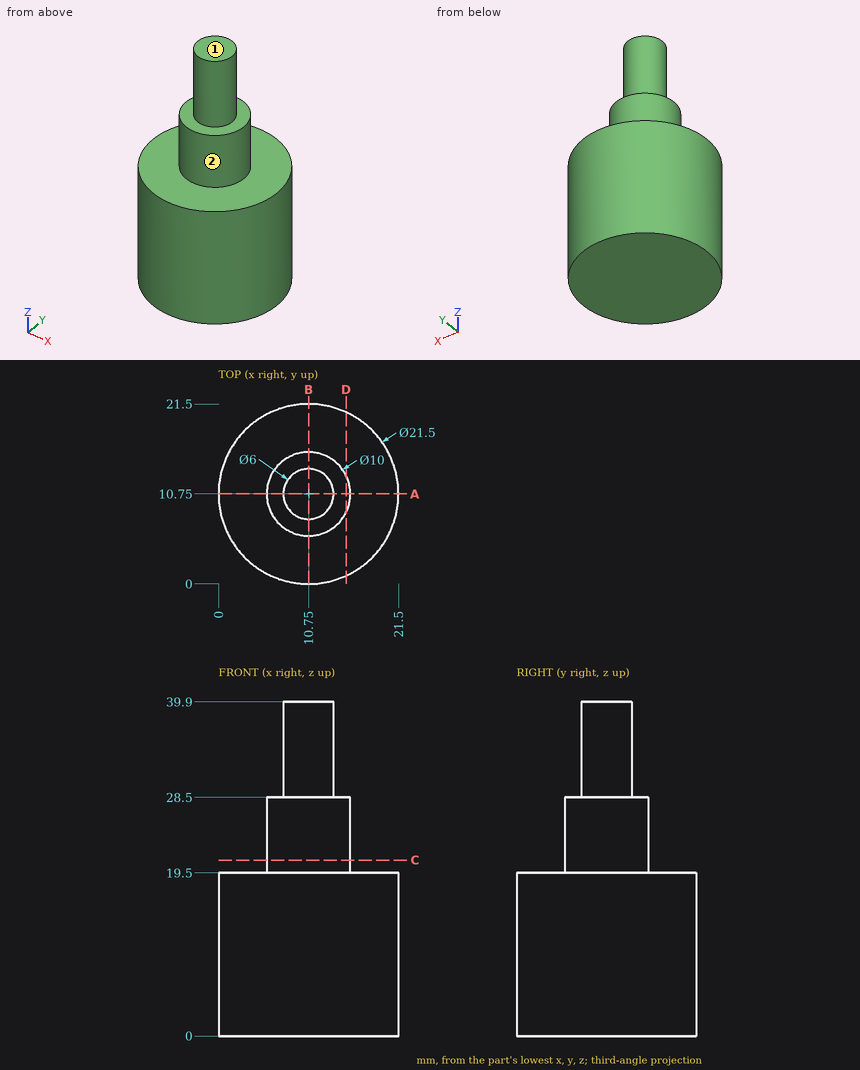
Design review of the part shown in the three views and the two pictorial views. Dimensions are in mm from the part's minimum x, y and z. A direction names the side the tool comes from. Give positions to 0.01 mm unless a question says otherwise; leave off trailing zeros. Loops run counter-clockwise (first coordinate to the right, second up) from the corner with the lowest first, then second, coordinate; pieces in that order, holes last. Notation, with made-up numbers: M 55,51.25 L 90,51.25 A24 ccw 90,65.25 Z; hole C -7,-16 d2. An arc over 180 degrees is marked long. Put each result on its own line as item: value. Start each with the question number.
(1) Add section D-D, the plane x = 15.25. Write out the cut boundary in (y, z).
(2) Wall thickness on L1, parallel to Z at x = 20.5, y = 10.75; L2, parallel to Z at x = 13.5, y = 8.5; L3, parallel to Y at x = 10.75, z = 38: over which ranges is each line inside the solid? List them lowest first.
(3) Add section A-A, the plane y = 10.75. Write out the cut boundary in (x, z), then the cut area to 3 significant figures.
(4) Machinability: for the marked faces 1 and 2, which of the approach directions +Z, -Z, +X, -X, +Y, -Y give a long, thin tool a straight path to every point of the face, cutting with its end or side? Answer none if there is none.
(5) Add section C-C, the plane z = 21. Write out the cut boundary in (x, y), then the cut area to 3 significant figures.
(6) For pin 1 (3 mm diameter, centred on x = 17, z = 5, fed in from +Y); pin 2 (2 mm diameter, centred on x = 5, y = 13.5, fed in from +Z); pin 3 (1 mm diameter, centred on x = 7, z = 19, fed in from +Y); pin 4 (5 mm diameter, centred on y = 19, z = 28.5, fed in from -X), all flat-tipped, find the tip position at first contact; note any pin that passes through.
Result:
1. outline: M 0.99,0 L 20.51,0 L 20.51,19.5 L 12.93,19.5 L 12.93,28.5 L 8.57,28.5 L 8.57,19.5 L 0.99,19.5 Z
2. L1: z = 0 to 19.5
2. L2: z = 0 to 28.5
2. L3: y = 7.75 to 13.75
3. outline: M 0,0 L 21.5,0 L 21.5,19.5 L 15.75,19.5 L 15.75,28.5 L 13.75,28.5 L 13.75,39.9 L 7.75,39.9 L 7.75,28.5 L 5.75,28.5 L 5.75,19.5 L 0,19.5 Z
3. area: 578 mm^2
4. face 1: +Z, +X, -X, +Y, -Y
4. face 2: +Z
5. outline: C 10.75,10.75 d10
5. area: 78.5 mm^2
6. pin 1: stops at y = 20.39
6. pin 2: stops at z = 19.5
6. pin 3: stops at y = 21
6. pin 4: passes through
